Source: CAD feature listing. Evaluate the final solid. Frame: model axes, mm. A direction names the side the tool comes from. Round coordinates to 2 decimals unless told otherwise and drop trailing zeros. Order: outer loops, then holes, each group sorted by start corner. A loop starts at its lowest first (then second) coordinate and runs counter-clockwise, first axis right, second up. Notation, with made-up numbers: (17.5, 43.5) -> (33.5, 43.5) arc R16 ccw to (33.5, 69.5) -> close; hole circle Ø11 at (-36, 45.5). An arc over 180 degrees is marked (long way). One line per item, written item: value. Start each with the question number.
1) Section C-C (y = -1). Return the cut outline in (x, z), and give its area (3 significant figures).
2) Section A-A (x = 32). Return the cut outline in (y, z).
3) Pin query (flat end, axial travel): P1, Ø4.5, axis at y = 9.5, z = 17.5, coming from the -X side; P2, Ø5.5, axis at x = -42.5, z = 13, coming from the -Y side; P3, Ø15, axis at x = -42.5, z = 21.5, coming from the +Y side. Return the tip coordinate at first contact, or that it passes through.
4) Ray query, L1, parallel to X at y = 9.8, z = 16.5; L2, parallel to Y at x = 31, z = 12; L3, parallel to Z at x = -23, y = -6.5. Return the intervals inside material, ascending.
5) Section D-D (x = -7). Return the cut outline in (y, z), and give its area (3 significant figures).
6) Section B-B (y = 9). Return the cut outline in (x, z).
7) Reachability of faces 1 (the face through (-35.936, -9.528, 21.032)), 2 (the face through (41.5, -7.5, 14.8)), 3 (the face through (29.57, 9.53, 28.4)) from +Z, -Z, +X, -X, +Y, -Y: full face, straight path, thin tool, end or side. Return the list, or none.
8) Mould query, pull axis Y, two halves, no side actions, for faces 4 (the face through (45, -10, 24)), 5 (the face through (-38.33, 6.9, 4.57)), 6 (the face through (30, -15, 2)). Classes: pulls with the +Y half, pulls with the -Y half, needs draft (parallel to the pull), parting line crosses it, or undercut.
```python
from build123d import *

# Parameters (mm, degrees)
SKETCH1_W                = 100
SKETCH1_H                = 30
BOSS_EXTRUDE1_DEPTH      = 4
SKETCH2_W                = 21
SKETCH2_H                = 4
BOSS_EXTRUDE2_DEPTH      = 25
CHAMFER1_SIZE            = 10
CHAMFER1_OF_MIRROR1_SIZE = 10
MIRROR2_START            = -11.5
MIRROR2_DEPTH            = 4
MIRROR2_START_2          = 7.5
MIRROR2_2_DEPTH          = 4
CUT_EXTRUDE1_DEPTH       = 64.586555183
FILLET1_R                = 10
FILLET2_R                = 2
CUT_EXTRUDE2_DEPTH       = 58.879184626


# Read off the part's stored shape, not the designer's step: Mirror2
with BuildPart() as part:
    # Sketch1 → Boss-Extrude1 (new body)
    with BuildSketch(Plane.XY):
        Rectangle(SKETCH1_W, SKETCH1_H)
    extrude(amount=BOSS_EXTRUDE1_DEPTH)

    # Sketch2 → Boss-Extrude2 (add)
    with BuildSketch(Plane.XY.offset(4)):
        with Locations((-39.5, -9.5)):
            Rectangle(SKETCH2_W, SKETCH2_H)
    boss_extrude2 = extrude(amount=BOSS_EXTRUDE2_DEPTH)

    # Chamfer1
    chamfer1_edges = [part.edges().sort_by_distance(p)[0] for p in [
        (-50, -9.5, 29),
    ]]
    chamfer(chamfer1_edges, length=CHAMFER1_SIZE)

    # Mirror1: Boss-Extrude2 across plane
    add(boss_extrude2.mirror(Plane.ZX))

    # Chamfer1 of Mirror1
    chamfer1_of_mirror1_edges = [part.edges().sort_by_distance(p)[0] for p in [
        (-50, 9.5, 29),
    ]]
    chamfer(chamfer1_of_mirror1_edges, length=CHAMFER1_OF_MIRROR1_SIZE)

    # Mirror2 outline → Mirror2 (add)
    with BuildSketch(Plane(origin=(0, 0, 0), x_dir=(1, 0, 0), z_dir=(0, 1, 0)).offset(MIRROR2_START)):
        Polygon((50, -19), (50, -4), (29, -4), (29, -29), (40, -29), align=None)
    extrude(amount=MIRROR2_DEPTH)

    # Mirror2 2 outline → Mirror2 2 (add)
    with BuildSketch(Plane(origin=(0, 0, 0), x_dir=(1, 0, 0), z_dir=(0, 1, 0)).offset(MIRROR2_START_2)):
        Polygon((50, -19), (50, -4), (29, -4), (29, -29), (40, -29), align=None)
    extrude(amount=MIRROR2_2_DEPTH)

    # Sketch3 → Cut-Extrude1 (cut, through all)
    with BuildSketch(Plane.XZ.offset(11.5)):
        with BuildLine():
            Line((-40.673413361, 18.935045716), (-37.5, 23.070718527))
            Line((-37.5, 23.070718527), (-34.326586639, 18.935045716))
            ThreePointArc((-34.326586639, 18.935045716), (-37.5, 12.5), (-40.673413361, 18.935045716))
        make_face()
    cut_extrude1 = extrude(amount=-CUT_EXTRUDE1_DEPTH, mode=Mode.SUBTRACT)

    # Mirror4: Cut-Extrude1 across plane
    add(cut_extrude1.mirror(Plane(origin=(0, 0, 0), x_dir=(0, 0, 1), z_dir=(1, 0, 0))), mode=Mode.SUBTRACT)

    # Fillet1
    # the kernel refuses this fillet: 10 mm, written as the material it takes off along each edge
    with BuildSketch(Plane(origin=(50, 15, -25), x_dir=(-1, 0, 0), z_dir=(0, 0, 1)), Plane(origin=(-50, 15, -25), x_dir=(0, -1, 0), z_dir=(0, 0, 1))) as fillet1_piece_1:
        with BuildLine():
            CenterArc((FILLET1_R, FILLET1_R), FILLET1_R, 180, 90)
            Line((0, FILLET1_R), (0, 0))
            Line((0, 0), (FILLET1_R, 0))
        make_face()
    extrude(amount=54, mode=Mode.SUBTRACT)
    with BuildSketch(Plane(origin=(50, -15, -25), x_dir=(-1, 0, 0), z_dir=(0, 0, 1)), Plane(origin=(-50, -15, -25), x_dir=(0, 1, 0), z_dir=(0, 0, 1))) as fillet1_piece_2:
        with BuildLine():
            CenterArc((FILLET1_R, -FILLET1_R), FILLET1_R, 90, 90)
            Line((0, -FILLET1_R), (0, 0))
            Line((0, 0), (FILLET1_R, 0))
        make_face()
    extrude(amount=54, mode=Mode.SUBTRACT)

    # Fillet2
    fillet2_edges = [part.edges().sort_by_distance(p)[0] for p in [
        (38.299671038, 11.5, 4),
        (-38.299671038, 11.5, 4),
        (-38.299671038, -11.5, 4),
        (38.299671038, -11.5, 4),
        (-29, -9.5, 4),
        (-39.341229183, -7.5, 4),
        (-29, -9.5, 29),
        (-40, -9.5, 29),
        (-29, 9.5, 29),
        (-29, 9.5, 4),
        (-39.341229183, 7.5, 4),
        (-40, 9.5, 29),
        (29, 9.5, 4),
        (39.341229183, 7.5, 4),
        (29, 9.5, 29),
        (40, 9.5, 29),
        (29, -9.5, 29),
        (29, -9.5, 4),
        (39.341229183, -7.5, 4),
        (40, -9.5, 29),
    ]]
    fillet(fillet2_edges, radius=FILLET2_R)

    # Sketch4 → Cut-Extrude2 (cut, through all)
    with BuildSketch(Plane.XY.offset(4)):
        Polygon((-15, 15), (15, 15), (21.062177826, 15), (15, 11.5), (-15, 11.5), (-21.062177826, 15), align=None)
    cut_extrude2 = extrude(amount=-CUT_EXTRUDE2_DEPTH, mode=Mode.SUBTRACT)

    # Mirror5: Cut-Extrude2 across plane
    add(cut_extrude2.mirror(Plane.ZX), mode=Mode.SUBTRACT)


solid = part.part
```
Findings:
1. outline: (-50, 0) -> (50, 0) -> (50, 4) -> (-50, 4) -> close
1. area: 400 mm2
2. outline: (-15, 0) -> (15, 0) -> (15, 4) -> (13.5, 4) arc R2 cw to (11.5, 6) -> (11.5, 29) -> (7.5, 29) -> (7.5, 6) arc R2 cw to (5.5, 4) -> (-5.5, 4) arc R2 cw to (-7.5, 6) -> (-7.5, 29) -> (-11.5, 29) -> (-11.5, 6) arc R2 cw to (-13.5, 4) -> (-15, 4) -> close
3. P1: x = -49.68
3. P2: y = -11.5
3. P3: y = 11.5
4. L1: -48.77 to -41.5, -33.5 to -29, 29 to 33.5, 41.5 to 48.77
4. L2: -11.5 to -7.5, 7.5 to 11.5
4. L3: 0 to 4
5. outline: (-11.5, 0) -> (11.5, 0) -> (11.5, 4) -> (-11.5, 4) -> close
5. area: 92.0 mm2
6. outline: (-49.17, 0) -> (49.17, 0) -> (49.17, 19.83) -> (40.59, 28.41) arc R2 ccw to (39.17, 29) -> (31, 29) arc R2 ccw to (29, 27) -> (29, 6) arc R2 cw to (27, 4) -> (-27, 4) arc R2 cw to (-29, 6) -> (-29, 27) arc R2 ccw to (-31, 29) -> (-39.17, 29) arc R2 ccw to (-40.59, 28.41) -> (-49.17, 19.83) -> close; hole (-40.67, 18.94) arc R4 ccw (long way) to (-34.33, 18.94) -> (-37.5, 23.07) -> close; hole (34.33, 18.94) arc R4 ccw (long way) to (40.67, 18.94) -> (37.5, 23.07) -> close
7. face 1: +Y, -Y
7. face 2: +Z, +X, -X
7. face 3: +Z, +Y, -Y
8. face 4: needs draft
8. face 5: undercut
8. face 6: pulls with the -Y half
